Here's the drawing with two shaded views (mm, measured from the low corner). I have some questions. Give positions to 0.01 mm unless a question says otherwise; leave off trailing zeros. Order: outer loops, then holes, each group sorted by start corner. A loop starts at its lowest first (then second) coordinate and runs counter-clockwise, first axis right, second up. Notation, with made-up numbers: M 75.25,68 L 124.25,68 A31 ccw 124.25,102 Z; hole C 12,-4.5 d11. An arc over 180 degrees is marked long. Write each question's results on one line, items separated by ' | '.
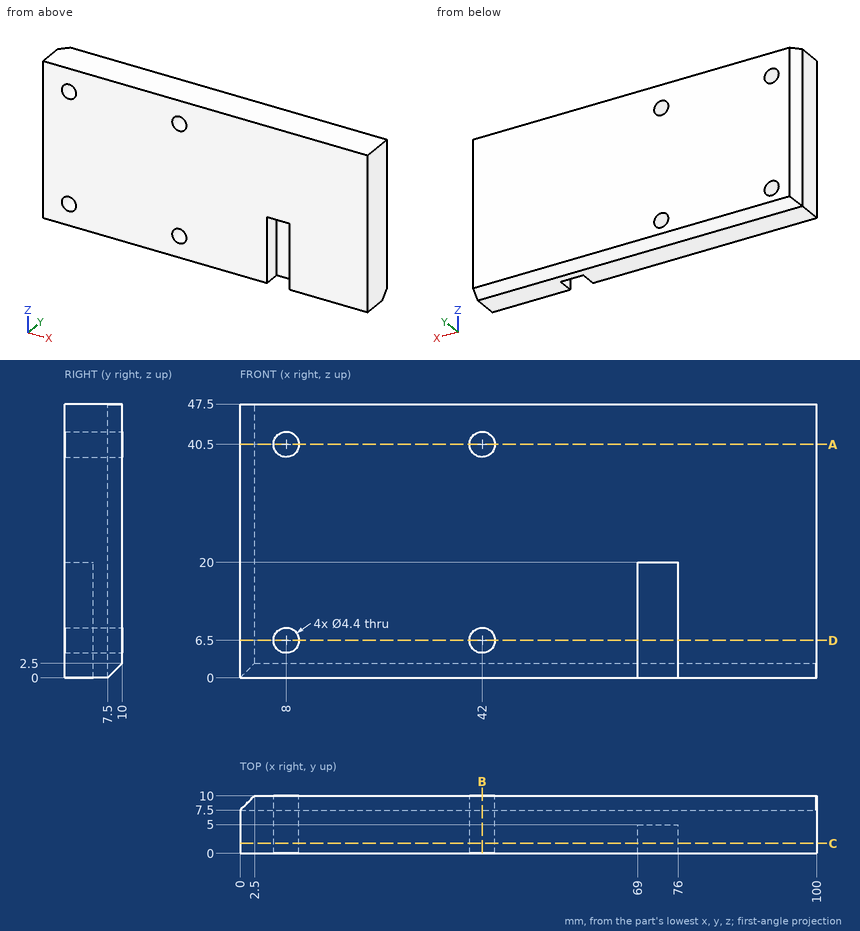
(1) Will these pins go through, and if not, where does the flat tip stop? P1, Ø3.5, axis at x = 8, z = 40.5, coming from the +Y side; P2, Ø5.5, axis at x = 72, z = 7, coming from the -Y side.
Data:
P1: passes through | P2: stops at y = 5
(2) I need wall thicknesses on L1, parallel to Z at x = 8, y = 5; L2, parallel to X at y = 4, z = 39; L3, parallel to X at y = 2.5, z = 41.5. Which ranges of each line are inside material? Lowest first, please. Write a range as from..to.
Data:
L1: z = 0..4.3, 8.7..38.3, 42.7..47.5 | L2: x = 0..6.39, 9.61..40.39, 43.61..100 | L3: x = 0..6.04, 9.96..40.04, 43.96..100
(3) Imagine slicing it at D-D, the plane z = 6.5. Write out the boundary of the cut face in (x, y).
Data:
outline: M 0,0 L 5.8,0 L 5.8,10 L 2.5,10 L 0,7.5 Z; M 10.2,0 L 39.8,0 L 39.8,10 L 10.2,10 Z; M 44.2,0 L 69,0 L 69,5 L 76,5 L 76,0 L 100,0 L 100,10 L 44.2,10 Z
(4) Imagine slicing it at C-C, the plane y = 1.75. Write out the boundary of the cut face in (x, z), plus the area to 3 significant figures.
Data:
outline: M 0,0 L 69,0 L 69,20 L 76,20 L 76,0 L 100,0 L 100,47.5 L 0,47.5 Z; hole C 8,6.5 d4.4; hole C 8,40.5 d4.4; hole C 42,6.5 d4.4; hole C 42,40.5 d4.4 | area: 4,550 mm2
(5) Imagine slicing it at A-A, the plane z = 40.5. Write out the boundary of the cut face in (x, y), plus the area to 3 significant figures.
Data:
outline: M 0,0 L 5.8,0 L 5.8,10 L 2.5,10 L 0,7.5 Z; M 10.2,0 L 39.8,0 L 39.8,10 L 10.2,10 Z; M 44.2,0 L 100,0 L 100,10 L 44.2,10 Z | area: 909 mm2
(6) Imagine slicing it at B-B, the plane x = 42. Write out the boundary of the cut face in (y, z), plus the area to 3 significant figures.
Data:
outline: M 0,0 L 7.5,0 L 10,2.5 L 10,4.3 L 0,4.3 Z; M 0,8.7 L 10,8.7 L 10,38.3 L 0,38.3 Z; M 0,42.7 L 10,42.7 L 10,47.5 L 0,47.5 Z | area: 384 mm2
